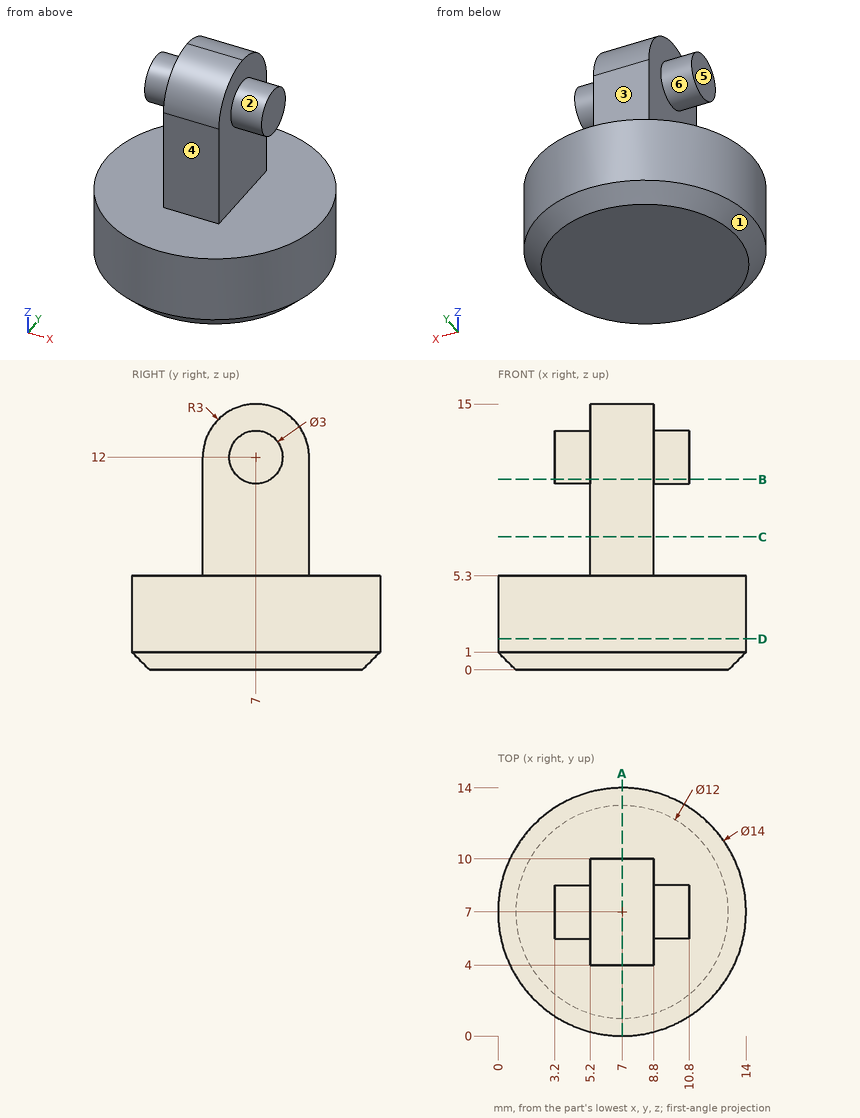
Part print with two shaded views. Sizes in mm from the minimum x, y, z corner. A direction names the side the tool comes from. Coordinates: 2 decimals unless noted, no trailing zeros. Write each loop counter-clockwise with the first axis right and the second up, starting at its lowest first coordinate (ties: lowest second). Pieces come first, ordered by that corner, then holes. Notation, with made-up numbers: (36.5, -32) - (50.5, -32) arc R28 ccw to (50.5, -9) - close; hole circle Ø2 at (4, 87.5). An arc over 180 degrees is marked (long way). Use a Markdown table: item, result. Add a question column.
Item 1: Drill centre lines: line 1 along X through (y, z) = (8.25, 7.5); line 2 along X through (y, z) = (6, 12.5); line 3 along Z through (x, y) = (2.75, 9.25). Where is each one in solid material? Low to high.
Item 2: Two-plate mould, pull along Z, no slides. Class the marked faces 1, 2 and 3: pulls with the +Z half, pulls with the -Z half, needs draft (parallel to the pull), parting line crosses it, or undercut.
Item 3: Band-saw the part on A-A, the plane x = 7. Write the cut outline in (y, z), and give its area (3 significant figures).
Item 4: Band-saw the part on B-B, the plane z = 10.75. Write the cut outline in (x, y).
Item 5: 3-axis set-ups, long thin cutter, end or side, ignore diameter. For the marked faces 4, 5 and 6: which of +Z, -Z, +X, -X, +Y, -Y reach the whole face in a straight line?
Item 6: Band-saw the part on D-D, the plane z = 1.75. Write the cut outline in (x, y).
Item 7: Band-saw the part on C-C, the plane z = 7.5. Write the cut outline in (x, y), and give its area (3 significant figures).
Item 8: Drop flat-ended pins along their axis: pin 1 (3 mm diameter, centred on x = 7, z = 7.5, fed in from +Y); pin 2 (3.5 mm diameter, centred on y = 7.5, z = 11.5, fed in from +X); pin 3 (5 mm diameter, centred on y = 7.5, z = 12, fed in from -X). Give the stop position or say it passes through.
A:
| question | item | result |
|---|---|---|
| 1 | line 1 | x = 5.2 to 8.8 |
| 1 | line 2 | x = 3.2 to 10.8 |
| 1 | line 3 | z = 0 to 5.3 |
| 2 | face 1 | pulls with the -Z half |
| 2 | face 2 | undercut |
| 2 | face 3 | needs draft |
| 3 | outline | (0, 1) - (1, 0) - (13, 0) - (14, 1) - (14, 5.3) - (10, 5.3) - (10, 12) arc R3 ccw to (4, 12) - (4, 5.3) - (0, 5.3) - close |
| 3 | area | 128 mm² |
| 4 | outline | (3.2, 6.17) - (5.2, 6.17) - (5.2, 4) - (8.8, 4) - (8.8, 6.17) - (10.8, 6.17) - (10.8, 7.83) - (8.8, 7.83) - (8.8, 10) - (5.2, 10) - (5.2, 7.83) - (3.2, 7.83) - close |
| 5 | face 4 | +Z, +X, -X, -Y |
| 5 | face 5 | +Z, -X, +Y, -Y |
| 5 | face 6 | -X |
| 6 | outline | circle Ø14 at (7, 7) |
| 7 | outline | (5.2, 4) - (8.8, 4) - (8.8, 10) - (5.2, 10) - close |
| 7 | area | 21.6 mm² |
| 8 | pin 1 | stops at y = 10 |
| 8 | pin 2 | stops at x = 10.8 |
| 8 | pin 3 | stops at x = 3.2 |
